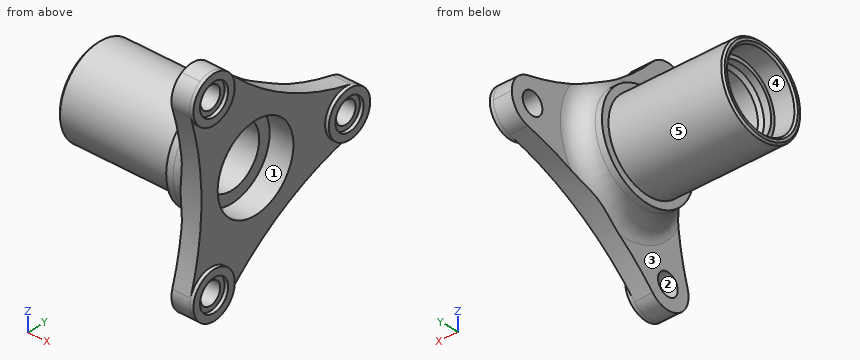
```python
from build123d import *

# Parameters (mm, degrees)
CHAMFER1_SIZE       = 1
FILLET1_R           = 10
SKETCH2_R           = 6
CUT_EXTRUDE1_DEPTH  = 30
BOSS_EXTRUDE1_START = 2
SKETCH3_R           = 12.6
SKETCH3_R_2         = 8.6
BOSS_EXTRUDE1_DEPTH = 2


with BuildPart() as part:
    # Sketch1 → Revolve1 (revolve)
    with BuildSketch(Plane.XY, mode=Mode.PRIVATE) as revolve1_sk:
        Polygon((0, 24), (62.5, 24), (62.5, 28), (76.2, 28), (76.2, 67.6), (86.2, 67.6), (86.2, 23.1), (73.2, 23.1), (73.2, 16.75), (17.45, 16.75), (15.7, 18.5), (11.8, 18.5), (11.8, 20.6), (0, 20.6), align=None)
    revolve(revolve1_sk.sketch.rotate(Axis((0, 0, 0), (1, 0, 0)), 90), axis=Axis((0, 0, 0), (1, 0, 0)))

    # Chamfer1
    chamfer1_edges = [part.edges().sort_by_distance(p)[0] for p in [
        (0, 0, -24),
        (0, 0, -20.6),
    ]]
    chamfer(chamfer1_edges, length=CHAMFER1_SIZE)

    # Fillet1
    fillet1_edges = [part.edges().sort_by_distance(p)[0] for p in [
        (76.2, 0, -28),
    ]]
    fillet(fillet1_edges, radius=FILLET1_R)

    # Sketch2 → Cut-Extrude1 (cut)
    with BuildSketch(Plane(origin=(86.2, 0, 0), x_dir=(0, 0, -1), z_dir=(1, 0, 0))):
        with BuildLine():
            ThreePointArc((-58.543317297, -33.799999998), (-60.092446992, -25.63392436), (-56.219136733, -18.279873653))
            ThreePointArc((-56.219136733, -18.279873653), (-28.550320514, 16.483535234), (-12.278733405, 57.827137417))
            ThreePointArc((-12.278733405, 57.827137417), (-7.846593801, 64.858547851), (0, 67.6))
            ThreePointArc((0, 67.6), (-58.543317295, 33.800000001), (-58.543317297, -33.799999998))
        make_face()
        with BuildLine():
            ThreePointArc((67.6, 0), (47.800418408, 47.800418408), (0, 67.6))
            ThreePointArc((0, 67.6), (7.846593801, 64.858547851), (12.278733405, 57.827137417))
            ThreePointArc((12.278733405, 57.827137417), (28.550320514, 16.483535234), (56.219136733, -18.279873653))
            ThreePointArc((56.219136733, -18.279873653), (60.092446945, -25.633924049), (58.543317611, -33.799999453))
            ThreePointArc((58.543317611, -33.799999453), (65.296585939, -17.496167144), (67.6, 0))
        make_face()
        with BuildLine():
            ThreePointArc((-43.940403329, -39.547263763), (-52.245853192, -39.22462349), (-58.543317297, -33.799999998))
            ThreePointArc((-58.543317297, -33.799999998), (3.14e-07, -67.6), (58.543317611, -33.799999453))
            ThreePointArc((58.543317611, -33.799999453), (52.245853485, -39.224623374), (43.940403329, -39.547263763))
            ThreePointArc((43.940403329, -39.547263763), (0, -32.967070468), (-43.940403329, -39.547263763))
        make_face()
        with Locations((47.631397208, -27.5)):
            Circle(SKETCH2_R)
        with Locations((-47.631397208, -27.5)):
            Circle(SKETCH2_R)
        with Locations((0, 55)):
            Circle(SKETCH2_R)
    extrude(amount=-CUT_EXTRUDE1_DEPTH, mode=Mode.SUBTRACT)

    # Sketch3 → Boss-Extrude1 (add)
    # profile 1 of 3: a face of its own
    with BuildSketch(Plane(origin=(86.2, 0, 0), x_dir=(0, 0, -1), z_dir=(1, 0, 0)).offset(BOSS_EXTRUDE1_START)):
        with Locations((0, 55)):
            Circle(SKETCH3_R)
        with Locations((0, 55)):
            Circle(SKETCH3_R_2, mode=Mode.SUBTRACT)
    # profile 2 of 3: a face of its own
    with BuildSketch(Plane(origin=(86.2, 0, 0), x_dir=(0, 0, -1), z_dir=(1, 0, 0)).offset(BOSS_EXTRUDE1_START)):
        with Locations((47.631397208, -27.5)):
            Circle(SKETCH3_R)
        with Locations((47.631397208, -27.5)):
            Circle(SKETCH3_R_2, mode=Mode.SUBTRACT)
    # profile 3 of 3: a face of its own
    with BuildSketch(Plane(origin=(86.2, 0, 0), x_dir=(0, 0, -1), z_dir=(1, 0, 0)).offset(BOSS_EXTRUDE1_START)):
        with Locations((-47.631397208, -27.5)):
            Circle(SKETCH3_R)
        with Locations((-47.631397208, -27.5)):
            Circle(SKETCH3_R_2, mode=Mode.SUBTRACT)
    extrude(amount=-BOSS_EXTRUDE1_DEPTH)


solid = part.part
```
Geometry check sheet. Reference: the model listing, model coordinates, mm. Face numbers are marked on the shaded views. A direction names the side the tool comes from. Coordinates: 2 decimals unless noted, no trailing zeros. Write each loop counter-clockwise with the first axis right and the second up, starting at its lowest first coordinate (ties: lowest second). Pieces come first, ordered by that corner, then holes. Notation, with made-up numbers: M -39.75,-27 L -31.75,-27 A16 cw -31.75,-13 Z; hole C 35.25,63.5 d9. An arc over 180 degrees is marked long. Use one line per item in the form item = value. Start each with the question number.
1) Release check for a two-part mould opening along Z. For the marked faces 3, 4 and 5 record: pulls with the +Z half, pulls with the -Z half, needs draft (parallel to the pull), parting line crosses it, or undercut.
2) Section check A-A on y = 52. Enter the section's corners in (x, z).
3) Thickness scan on probe 1 along Y at (x, z) = (81, 0); probe 2 along Z at (x, y) = (80, -27); probe 3 along Y at (x, z) = (13, 0). Record the ranges inside material, lowest first. Write a range as from..to.
4) Section check B-B on z = -51.5. Enter the section's corners in (x, y).
5) Set-up check for the marked faces 1 and 2: record each of +Z, -Z, +X, -X, +Y, -Y from which the full face is reachable in a straight line by a thin tool's end or side.
6) Go/stop test with flat-tipped pins: pin 1 Ø8 at (x, z) = (73, 42.5) entering from -Y; pin 2 Ø23 at (y, z) = (0, 6) entering from +X; pin 3 Ø22.5 at (y, z) = (55, 0) entering from -X; pin 4 Ø1 at (y, z) = (-0.5, 22.5) entering from -X. Record where each tip stops, or that it passes through.
7) Section check C-C on x = 60. Enter the section's corners in (y, z), and give its area (3 significant figures).
Responses:
q1.face_3 = needs draft
q1.face_4 = undercut
q1.face_5 = parting line crosses it
q2.outline = M 76.2,-13.74 L 86.2,-13.74 L 86.2,-12.24 L 88.2,-12.24 L 88.2,-8.06 L 86.2,-8.06 L 86.2,-5.2 L 76.2,-5.2 Z; M 76.2,5.2 L 86.2,5.2 L 86.2,8.06 L 88.2,8.06 L 88.2,12.24 L 86.2,12.24 L 86.2,13.74 L 76.2,13.74 Z
q3.probe_1 = -32.97..-23.1, 23.1..49, 61..67.6
q3.probe_2 = -60.22..-53.61, -41.65..41.65, 53.61..60.22
q3.probe_3 = -24..-18.5, 18.5..24
q4.outline = M 76.2,-39.49 L 88.2,-39.49 L 88.2,-35.18 L 86.2,-35.18 L 86.2,-32.09 L 76.2,-32.09 Z; M 76.2,-22.91 L 86.2,-22.91 L 86.2,-19.82 L 88.2,-19.82 L 88.2,-15.51 L 86.2,-15.51 L 86.2,-13.69 L 76.2,-13.69 Z
q5.face_1 = +X
q5.face_2 = +X, -X
q6.pin_1 = -39.8
q6.pin_2 = 73.2
q6.pin_3 = 76.2
q6.pin_4 = 0
q7.outline = C 0,0 d48; hole C 0,0 d33.5
q7.area = 928 mm2
